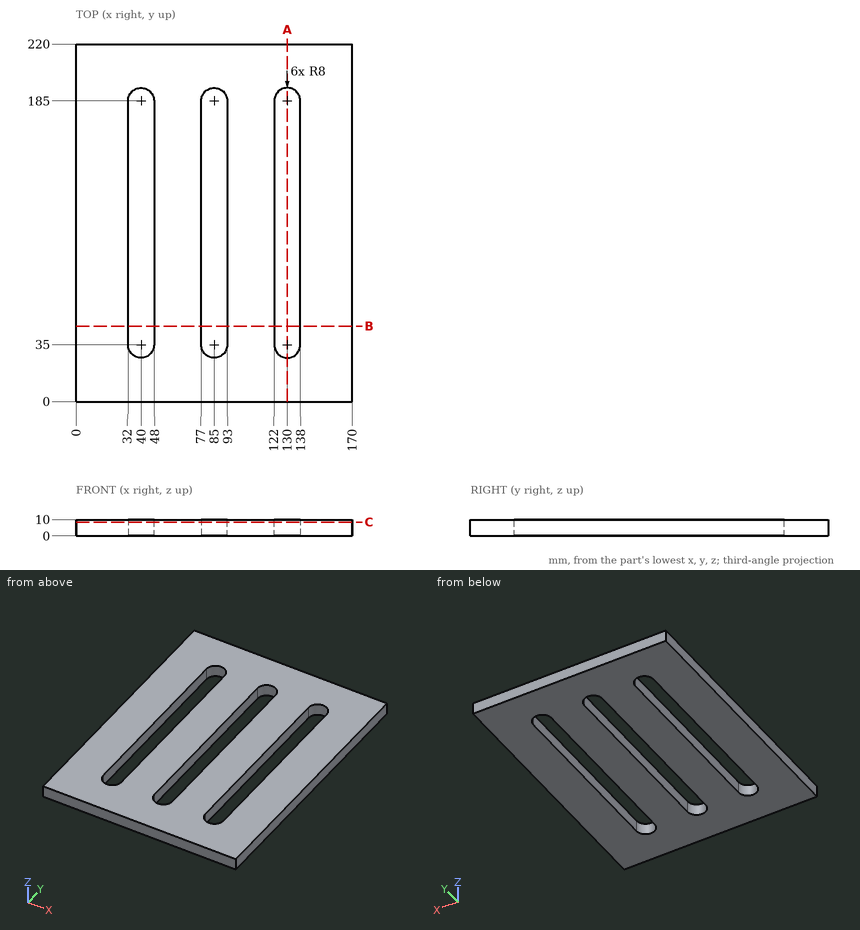
Design review of the part shown in the three views and the two pictorial views. Dimensions are in mm from the part's minimum x, y and z. Round coordinates to 2 decimals unless told otherwise and drop trailing zeros. Loops run counter-clockwise (first coordinate to the right, second up) from the corner with the lowest first, then second, coordinate; pieces in that order, holes last. Notation, with made-up numbers: (-10, 17) - (-1, 17) arc R28 cw to (-1, 39) - close; hole circle Ø7 at (-22.5, 2). An arc over 180 degrees is marked (long way). Write each question's results on one line, items separated by ' | '. Start each with the question number.
Q1. Take a section at A-A on x = 130. Give the boundary of the cut face in (y, z), plus the area to 3 significant figures.
Q2. Wall thickness on line 1 along X through (y, z) = (50.5, 1.5); line 2 along Y through (x, z) = (78.5, 7.75): over which ranges is each line inside the solid? List them lowest first. Write a range as [from, to].
Q3. Take a section at C-C on z = 8.5. Give the boundary of the cut face in (x, y).
Q4. Take a section at B-B on y = 46.5. Give the boundary of the cut face in (x, z), plus the area to 3 significant figures.
Data:
1) outline: (0, 0) - (27, 0) - (27, 10) - (0, 10) - close; (193, 0) - (220, 0) - (220, 10) - (193, 10) - close | area: 540 mm²
2) line 1: x = [0, 32], [48, 77], [93, 122], [138, 170] | line 2: y = [0, 30.34], [189.66, 220]
3) outline: (0, 0) - (170, 0) - (170, 220) - (0, 220) - close; hole (32, 35) arc R8 ccw to (48, 35) - (48, 185) arc R8 ccw to (32, 185) - close; hole (77, 35) arc R8 ccw to (93, 35) - (93, 185) arc R8 ccw to (77, 185) - close; hole (122, 35) arc R8 ccw to (138, 35) - (138, 185) arc R8 ccw to (122, 185) - close
4) outline: (0, 0) - (32, 0) - (32, 10) - (0, 10) - close; (48, 0) - (77, 0) - (77, 10) - (48, 10) - close; (93, 0) - (122, 0) - (122, 10) - (93, 10) - close; (138, 0) - (170, 0) - (170, 10) - (138, 10) - close | area: 1,220 mm²
